Design review of the part shown in the three views and the two pictorial views. Dimensions are in mm from the part's minimum x, y and z. Coordinates: 2 decimals unless noted, no trailing zeros. Loops run counter-clockwise (first coordinate to the right, second up) from the corner with the lowest first, then second, coordinate; pieces in that order, holes last. Notation, with made-up numbers: (-36.5, -12) -> (-30.5, -12) arc R28 ccw to (-30.5, 19) -> close; hole circle Ø1 at (66, -35). An arc over 180 degrees is marked (long way). Use CSV: the item, a comma, the result in double quotes.
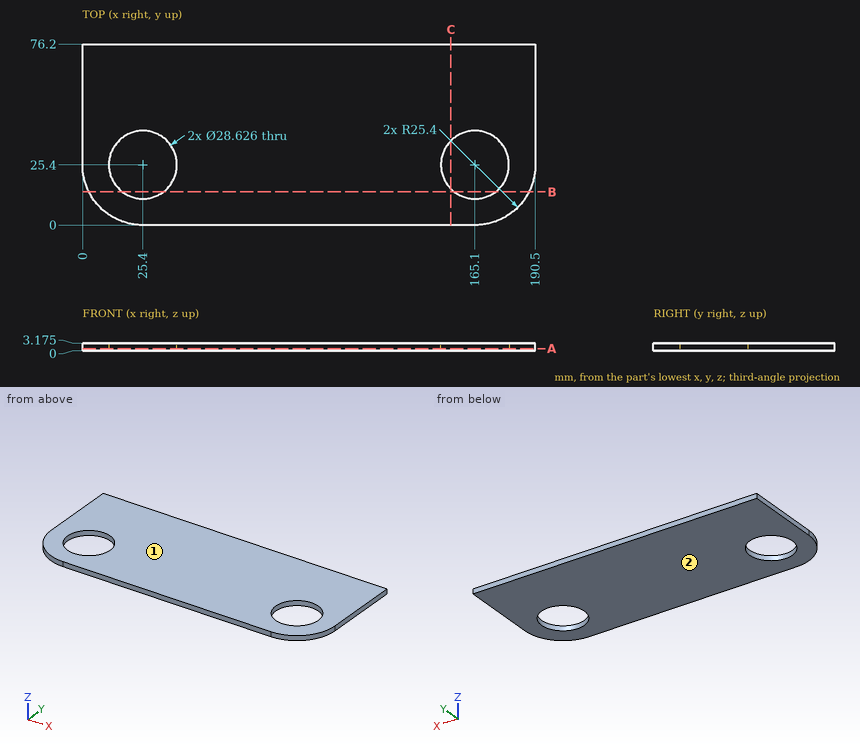
Item 1: Clearance check with a flat-ended pin moving along its axis: pin 1 (1 mm diameter, centred on x = 166.5, z = 1, fed in from -Y). State where the tip first meets the part, or that it passes through.
Checked values:
pin 1,"y = 0.02"
Item 2: Add section A-A (z = 0.9). Give the boundary of the cut face in (x, y), then the cut area to 3 significant figures.
Checked values:
outline,"(0, 25.4) arc R25.4 ccw to (25.4, 0) -> (165.1, 0) arc R25.4 ccw to (190.5, 25.4) -> (190.5, 76.2) -> (0, 76.2) -> close; hole circle Ø28.63 at (25.4, 25.4); hole circle Ø28.63 at (165.1, 25.4)"
area,"13,000 mm^2"
Item 3: Add section B-B (y = 14). Give the boundary of the cut face in (x, z) (1 decimal), then the cut area to 3 significant figures.
Checked values:
outline,"(2.7, 0) -> (16.7, 0) -> (16.7, 3.2) -> (2.7, 3.2) -> close; (34.1, 0) -> (156.4, 0) -> (156.4, 3.2) -> (34.1, 3.2) -> close; (173.8, 0) -> (187.8, 0) -> (187.8, 3.2) -> (173.8, 3.2) -> close"
area,"478 mm^2"
Item 4: Draft analysis for pull direction Z (two halves, no side actions). For the marked faces 1 and 2, state which applies: pulls with the +Z half, pulls with the -Z half, needs draft (parallel to the pull), parting line crosses it, or undercut.
Checked values:
face 1,"pulls with the +Z half"
face 2,"pulls with the -Z half"
Item 5: Add section C-C (x = 155). Give the boundary of the cut face in (y, z) (1 decimal).
Checked values:
outline,"(0, 0) -> (15.3, 0) -> (15.3, 3.2) -> (0, 3.2) -> close; (35.5, 0) -> (76.2, 0) -> (76.2, 3.2) -> (35.5, 3.2) -> close"
Item 6: To check wall thickness, follow line 1 along Y through (x, z) = (165.1, 2.05); line 2 along X through (y, z) = (35, 2.55) (1 decimal); line 3 along X through (y, z) = (26.5, 1.75). State the ranges of each line that lie inside material, in increasing order.
Checked values:
line 1,"0 to 11.09, 39.71 to 76.2"
line 2,"0 to 14.8, 36 to 154.5, 175.7 to 190.5"
line 3,"0 to 11.13, 39.67 to 150.83, 179.37 to 190.5"
